from build123d import *

# Parameters (mm, degrees)
SKETCH_2_R          = 9.5
SKETCH_2_R_2        = 11
EXTRUDE_1_DEPTH     = 6
CUT_EXTRUDE_1_DEPTH = 10
FILLET_1_R          = 25
SKETCH_4_R          = 2.75
CUT_EXTRUDE_2_DEPTH = 10
FILLET_2_R          = 15
FILLET_3_R          = 1


with BuildPart() as part:
    # 草图2 → 凸台-拉伸1 (new body)
    with BuildSketch(Plane(origin=(0, 0, 0), x_dir=(0, 0, -1), z_dir=(1, 0, 0))):
        Polygon((12.494318662, 71.640794729), (-72.751567756, -76.009411684), (-12.535755442, -411.712565336), (72.916857811, -263.704297543), align=None)
        with Locations((-40, -117)):
            Circle(SKETCH_2_R, mode=Mode.SUBTRACT)
        with Locations((25, -296.698729811)):
            Circle(SKETCH_2_R_2, mode=Mode.SUBTRACT)
        with Locations((0, -340)):
            Circle(SKETCH_2_R_2, mode=Mode.SUBTRACT)
        with Locations((-25, -43.301270189)):
            Circle(SKETCH_2_R_2, mode=Mode.SUBTRACT)
        with Locations((40, -222)):
            Circle(SKETCH_2_R, mode=Mode.SUBTRACT)
        Circle(SKETCH_2_R_2, mode=Mode.SUBTRACT)
    extrude(amount=EXTRUDE_1_DEPTH)

    # 草图3 → 切除-拉伸1 (cut)
    with BuildSketch(Plane(origin=(6, 0, 0), x_dir=(0, 0, -1), z_dir=(1, 0, 0))):
        with BuildLine():
            Line((-20.40575236, -141.278289439), (7.842954525, -298.764830322))
            ThreePointArc((7.842954525, -298.764830322), (-0.2344101, -310.373283308), (-11.842863085, -302.295918683))
            Line((-11.842863085, -302.295918683), (-40.09156997, -144.8093778))
            ThreePointArc((-40.09156997, -144.8093778), (-32.014205345, -133.200924814), (-20.40575236, -141.278289439))
        make_face()
        with BuildLine():
            Line((11.783440235, -37.201240644), (40.155401092, -194.665623401))
            ThreePointArc((40.155401092, -194.665623401), (32.087124724, -206.280394877), (20.472353248, -198.212118508))
            Line((20.472353248, -198.212118508), (-7.89960761, -40.747735751))
            ThreePointArc((-7.89960761, -40.747735751), (0.168668759, -29.132964275), (11.783440235, -37.201240644))
        make_face()
    extrude(amount=-CUT_EXTRUDE_1_DEPTH, mode=Mode.SUBTRACT)

    # 圆角1
    fillet_1_edges = [part.edges().sort_by_distance(p)[0] for p in [
        (3, -411.712565336, 12.535755442),
        (3, 71.640794729, -12.494318662),
    ]]
    fillet(fillet_1_edges, radius=FILLET_1_R)

    # 草图4 → 切除-拉伸2 (cut)
    with BuildSketch(Plane(origin=(6, 0, 0), x_dir=(0, 0, -1), z_dir=(1, 0, 0))):
        with Locations((-49.820508076, -46.291651246)):
            Circle(SKETCH_4_R)
        with Locations((-64.820508076, -72.27241336)):
            Circle(SKETCH_4_R)
        with Locations((-48.660254038, -64.282032303)):
            Circle(SKETCH_4_R)
        with Locations((48.660254038, -275.717967697)):
            Circle(SKETCH_4_R)
        with Locations((49.820508076, -293.708348754)):
            Circle(SKETCH_4_R)
        with Locations((64.820508076, -267.72758664)):
            Circle(SKETCH_4_R)
        Polygon((-66.650635095, -65.442286341), (-56.650635095, -48.121778265), (-47.990381057, -53.121778265), (-57.990381057, -70.442286341), align=None)
        Polygon((47.990381057, -286.878221735), (57.990381057, -269.557713659), (66.650635095, -274.557713659), (56.650635095, -291.878221735), align=None)
    extrude(amount=-CUT_EXTRUDE_2_DEPTH, mode=Mode.SUBTRACT)

    # 圆角2
    fillet_2_edges = [part.edges().sort_by_distance(p)[0] for p in [
        (3, -263.704297543, -72.916857811),
        (3, -76.009411684, 72.751567756),
    ]]
    fillet(fillet_2_edges, radius=FILLET_2_R)

    # 圆角3
    fillet_3_edges = [part.edges().sort_by_distance(p)[0] for p in [
        (3, -286.878221735, -47.990381057),
        (3, -269.557713659, -57.990381057),
        (3, -53.121778265, 47.990381057),
        (3, -70.442286341, 57.990381057),
    ]]
    fillet(fillet_3_edges, radius=FILLET_3_R)


solid = part.part
CAD build for the part. Positions are in the model's coordinates, mm. A direction names the side the tool comes from. Round coordinates to 2 decimals unless told otherwise and drop trailing zeros. Write each loop counter-clockwise with the first axis right and the second up, starting at its lowest first coordinate (ties: lowest second). Pieces come first, ordered by that corner, then holes. Notation, with made-up numbers: M -2,79.5 L 6,79.5 A22 ccw 6,94.5 Z; hole C 18.5,49 d10. An arc over 180 degrees is marked long. Use a Markdown table: item, result. Add a question column.
1. Slice it at D-D on x = 3.5. Give the number of separate pieces and of enclosed holes in the cut face, then the cut area to 3 significant figures.
2. Slice it at C-C on y = 0. Give the cut face in (x, z), then the cut area to 3 significant figures.
3. Slice it at A-A on z = 0. Give the cut face in (x, y).
4. Slice it at B-B on y = -150.5. Give the cut face in (x, z).
5. Drill centre lines: probe 1 along Z at (x, y) = (4, -62.5); probe 2 along Z at (x, y) = (0.5, -290); probe 3 along Z at (x, y) = (2.5, -279). Where is each one in solid material? Low to high.
6. Flat gauge pins, fed straight in: P1, Ø17, axis at y = -222, z = -40, coming from the -X side; P2, Ø1.5, axis at x = 4.5, y = -126, coming from the +Z side; P3, Ø7, axis at y = -293.71, z = -49.82, coming from the +X side. Where does each tip first touch, or does it go through?
7. 3-axis set-ups, long thin cutter, end or side, ignore diameter. For faces 1 (the face through (2.958, -322.613, -38.906)), 2 (the face through (3.042, -61.673, 52.927)): which of +Z, -Z, +X, -X, +Y, -Y reach the whole face in a straight line?
Reply:
| question | item | result |
|---|---|---|
| 1 | separate pieces | 1 |
| 1 | enclosed holes | 14 |
| 1 | area | 26,000 mm^2 |
| 2 | outline | M 0,-25.4 L 6,-25.4 L 6,-11 L 0,-11 Z; M 0,11 L 6,11 L 6,28.87 L 0,28.87 Z |
| 2 | area | 194 mm^2 |
| 3 | outline | M 0,-365 L 6,-365 L 6,-351 L 0,-351 Z; M 0,-329 L 6,-329 L 6,-310.33 L 0,-310.33 Z; M 0,-255.04 L 6,-255.04 L 6,-84.59 L 0,-84.59 Z; M 0,-29.16 L 6,-29.16 L 6,-11 L 0,-11 Z; M 0,11 L 6,11 L 6,25 L 0,25 Z |
| 4 | outline | M 0,-52.52 L 6,-52.52 L 6,-32.2 L 0,-32.2 Z; M 0,-11.88 L 6,-11.88 L 6,18.75 L 0,18.75 Z; M 0,39.07 L 6,39.07 L 6,59.39 L 0,59.39 Z |
| 5 | probe 1 | z = -36.66 to -16.34, 3.98 to 46.57, 50.75 to 53.4 |
| 5 | probe 2 | z = -53.4 to -33.73, -16.27 to -6.27, 14.05 to 34.37 |
| 5 | probe 3 | z = -52.54 to -4.3, 16.02 to 36.34 |
| 6 | P1 | passes through |
| 6 | P2 | stops at z = 63.92 |
| 6 | P3 | stops at x = 6 |
| 7 | face 1 | -Z, +X, -X, -Y |
| 7 | face 2 | +X, -X |
